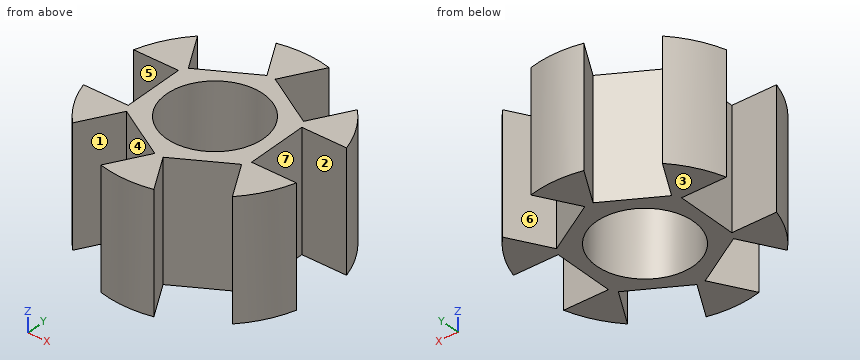
from build123d import *

# Parameters (mm, degrees)
SKETCH1_R           = 9.25
SKETCH1_R_2         = 4.05
BOSS_EXTRUDE1_DEPTH = 5
SKETCH2_W           = 5.15
SKETCH2_H           = 10
CUT_EXTRUDE3_DEPTH  = 4.1
CIRPATTERN1_COUNT   = 6


with BuildPart() as part:
    # Sketch1 → Boss-Extrude1 (new body, symmetric)
    with BuildSketch(Plane.XY):
        Circle(SKETCH1_R)
        Circle(SKETCH1_R_2, mode=Mode.SUBTRACT)
    extrude(amount=BOSS_EXTRUDE1_DEPTH, both=True)

    # Sketch2 → Cut-Extrude3 (cut)
    with BuildSketch(Plane(origin=(-9.25, -17.193061184, 0), x_dir=(0, -1, 0), z_dir=(1, 0, 0))):
        with Locations((-17.193061184, 0)):
            Rectangle(SKETCH2_W, SKETCH2_H)
    cut_extrude3 = extrude(amount=CUT_EXTRUDE3_DEPTH, mode=Mode.SUBTRACT)

    # CirPattern1: Cut-Extrude3 ×6 about axis
    cirpattern1_axis = Axis((0, 0, 0), (0, 0, 1))
    for i in range(1, CIRPATTERN1_COUNT):
        add(cut_extrude3.rotate(cirpattern1_axis, i * 360 / CIRPATTERN1_COUNT), mode=Mode.SUBTRACT)


solid = part.part
Work out the finished part from the listing and answer in its coordinate system (mm). Face numbers are marked on the shaded views. A direction names the side the tool comes from. Round coordinates to 2 decimals unless told otherwise and drop trailing zeros. Write each loop counter-clockwise with the first axis right and the second up, starting at its lowest first coordinate (ties: lowest second). Pieces come first, ordered by that corner, then holes.
1) The mould has two halves that part along Y. Classify the marked faces 1, 2 and 3: pulls with the +Y half, pulls with the -Y half, needs draft (parallel to the pull), parting line crosses it, or undercut.
2) Given pin 1 Ø4 at (x, z) = (7.5, 0.5) entering from +Y; pin 2 Ø1 at (y, z) = (7.5, -2.5) entering from -X; pin 3 Ø1.1 at (x, z) = (7.5, 2) entering from -Y; pin 4 Ø1 at (x, y) = (1.5, -0.5) entering from +Z, each flat-ended and moving along its own axis, determine where each tip first touches the part or whether it passes through.
3) A tool of negligible diameter and unlimited length cuts with its end or side. For the marked faces 4, 5, 6 and 7, from which of +Z, -Z, +X, -X, +Y, -Y can it reach the whole face along a straight path? Write none if from no direction.
4) A cutting plane is placed at D-D (y = -3.75). Give the vertices of the cut face in (x, z), plus the area to 3 significant figures.
5) A cutting plane is placed at C-C (z = 1). Give the vertices of the cut face in (x, y) (3 decimals), plus the area to 3 significant figures.
6) A cutting plane is placed at A-A (x = 0). Give the vertices of the cut face in (y, z), plus the area to 3 significant figures.
7) Straight lines are drawn through the part: line 1 (Y direction, x = 2, z = 4.25); line 2 (Y direction, x = 0, z = 0.5); line 3 (Y direction, x = -0.5, z = -0.5). For each, find the intervals that lie inside material, in ascending order.
8) A cutting plane is placed at B-B (y = 0). Give the vertices of the cut face in (x, z), plus the area to 3 significant figures.
Completed:
1. face 1: pulls with the -Y half
1. face 2: undercut
1. face 3: needs draft
2. pin 1: stops at y = 6.41
2. pin 2: stops at x = -1.65
2. pin 3: stops at y = -6.1
2. pin 4: passes through
3. face 4: +Z, -Z
3. face 5: +Z, -Z, -X
3. face 6: +Z, -Z, +Y
3. face 7: +Z, -Z, +X
4. outline: (-8.46, -5) - (-5.14, -5) - (-5.14, 5) - (-8.46, 5) - close; (-3.8, -5) - (-1.53, -5) - (-1.53, 5) - (-3.8, 5) - close; (1.53, -5) - (3.8, -5) - (3.8, 5) - (1.53, 5) - close; (5.14, -5) - (8.46, -5) - (8.46, 5) - (5.14, 5) - close
4. area: 112 mm2
5. outline: (-8.884, -2.575) arc R9.25 ccw to (-6.672, -6.407) - (-4.805, -3.173) - (-0.345, -5.748) - (-2.212, -8.982) arc R9.25 ccw to (2.212, -8.982) - (0.345, -5.748) - (4.805, -3.173) - (6.672, -6.407) arc R9.25 ccw to (8.884, -2.575) - (5.15, -2.575) - (5.15, 2.575) - (8.884, 2.575) arc R9.25 ccw to (6.672, 6.407) - (4.805, 3.173) - (0.345, 5.748) - (2.212, 8.982) arc R9.25 ccw to (-2.212, 8.982) - (-0.345, 5.748) - (-4.805, 3.173) - (-6.672, 6.407) arc R9.25 ccw to (-8.884, 2.575) - (-5.15, 2.575) - (-5.15, -2.575) - close; hole circle Ø8.1 at (0, 0)
5. area: 94.3 mm2
6. outline: (-9.25, -5) - (-4.05, -5) - (-4.05, 5) - (-9.25, 5) - close; (4.05, -5) - (9.25, -5) - (9.25, 5) - (4.05, 5) - close
6. area: 104 mm2
7. line 1: y = -9.03 to -8.61, -4.79 to -3.52, 3.52 to 4.79, 8.61 to 9.03
7. line 2: y = -9.25 to -4.05, 4.05 to 9.25
7. line 3: y = -9.24 to -6.02, -5.66 to -4.02, 4.02 to 5.66, 6.02 to 9.24
8. outline: (-5.15, -5) - (-4.05, -5) - (-4.05, 5) - (-5.15, 5) - close; (4.05, -5) - (5.15, -5) - (5.15, 5) - (4.05, 5) - close
8. area: 22.0 mm2
